Build history of the part. All positions in model axes, mm. A direction names the side the tool comes from. Give positions to 0.01 mm unless a question says otherwise; leave off trailing zeros. Order: outer loops, then holes, each group sorted by start corner. A loop starts at its lowest first (then second) coordinate and runs counter-clockwise, first axis right, second up. Notation, with made-up numbers: M -1.5,36 L 22.5,36 A31 ccw 22.5,71 Z; hole C 20,2 d1. An arc over 180 degrees is marked long. Use CSV: the item, a comma, the result in double quotes. Start each with the question number.
Item 1: Pin check, flat tip, straight feed: P1, Ø6.5, axis at x = 20.5, y = 3.5, coming from the +Z side. Stop position of the tip, or through.
Item 2: Which spindle directions (+Z, -Z, +X, -X, +Y, -Y) get a long thin tool onto all of the face, cutting with end or side? Do faces 4 (the flat face through (14, 29, 12)), 5 (the flat face through (4, 24, 7)), 6 (the cylindrical face through (-4, 38.07, 9.86)). Say none if no direction does.
Item 3: Band-saw the part on B-B on z = 16. Write the cut outline in (x, y).
Item 4: Two-plate mould, pull along Y, no slides. Class faces 1 (the flat face through (5, 26, 0)), 2 (the flat face through (14, -3, 10)), 3 (the flat face through (14, -10.5, 10)): pulls with the +Y half, pulls with the -Y half, needs draft (parallel to the pull), parting line crosses it, or undercut.
Item 5: Band-saw the part on D-D on y = 28. Write the cut outline in (x, z).
Item 6: Band-saw the part on A-A on x = 22. Write the cut outline in (y, z), plus the area to 3 significant figures.
Item 7: Wall check: line 1 along Y through (x, z) = (28.5, 17.5); line 2 along Y through (x, z) = (18, 10); line 3 along X through (y, z) = (14, 12.5). Give the ranges that are in metal, low to high.
Item 8: Band-saw the part on C-C on y = 21.5. Write the cut outline in (x, z), plus the area to 3 significant figures.
from build123d import *

# Parameters (mm, degrees)
SKETCH2_W           = 29
SKETCH2_H           = 5
BOSS_EXTRUDE2_DEPTH = 20
SKETCH3_W           = 8
SKETCH3_H           = 5
SKETCH3_W_2         = 29
SKETCH3_H_2         = 6
CUT_EXTRUDE1_DEPTH  = 5


with BuildPart() as part:
    # Sketch2 → Boss-Extrude2 (new body)
    with BuildSketch(Plane.XY):
        with BuildLine():
            ThreePointArc((-5.5, -5.5), (-4.035533906, -9.035533906), (-0.5, -10.5))
            Line((-0.5, -10.5), (29.5, -10.5))
            ThreePointArc((29.5, -10.5), (33.035533906, -9.035533906), (34.5, -5.5))
            Line((34.5, -5.5), (34.5, 34.5))
            ThreePointArc((34.5, 34.5), (33.035533906, 38.035533906), (29.5, 39.5))
            Line((29.5, 39.5), (-0.5, 39.5))
            ThreePointArc((-0.5, 39.5), (-4.035533906, 38.035533906), (-5.5, 34.5))
            Line((-5.5, 34.5), (-5.5, -5.5))
        make_face()
        Polygon((29, 6), (0, 6), (0, 24), (8, 24), (8, 29), (21, 29), (21, 24), (29, 24), align=None, mode=Mode.SUBTRACT)
        with Locations((14.5, -5.5)):
            Rectangle(SKETCH2_W, SKETCH2_H, mode=Mode.SUBTRACT)
        with Locations((14.5, 34.5)):
            Rectangle(SKETCH2_W, SKETCH2_H, mode=Mode.SUBTRACT)
    extrude(amount=BOSS_EXTRUDE2_DEPTH)

    # Sketch3 → Cut-Extrude1 (cut)
    with BuildSketch(Plane.XY.offset(20)):
        with Locations((4, 26.5)):
            Rectangle(SKETCH3_W, SKETCH3_H)
        with Locations((25, 26.5)):
            Rectangle(SKETCH3_W, SKETCH3_H)
        with Locations((14.5, 3)):
            Rectangle(SKETCH3_W_2, SKETCH3_H_2)
    extrude(amount=-CUT_EXTRUDE1_DEPTH, mode=Mode.SUBTRACT)


solid = part.part
Model answer:
1,P1,"stops at z = 15"
2,face 4,"+Z"
2,face 5,"+Z, -Z"
2,face 6,"+Z, -Z, -X, +Y"
3,outline,"M -5.5,-5.5 A5 ccw -0.5,-10.5 L 29.5,-10.5 A5 ccw 34.5,-5.5 L 34.5,34.5 A5 ccw 29.5,39.5 L -0.5,39.5 A5 ccw -5.5,34.5 Z; hole M 0,-8 L 29,-8 L 29,-3 L 0,-3 Z; hole M 0,0 L 29,0 L 29,29 L 0,29 Z; hole M 0,32 L 29,32 L 29,37 L 0,37 Z"
4,face 1,"needs draft"
4,face 2,"undercut"
4,face 3,"pulls with the -Y half"
5,outline,"M -5.5,0 L 8,0 L 8,15 L 0,15 L 0,20 L -5.5,20 Z; M 21,0 L 34.5,0 L 34.5,20 L 29,20 L 29,15 L 21,15 Z"
6,outline,"M -10.5,0 L -8,0 L -8,20 L -10.5,20 Z; M -3,0 L 6,0 L 6,15 L 0,15 L 0,20 L -3,20 Z; M 24,0 L 32,0 L 32,20 L 29,20 L 29,15 L 24,15 Z; M 37,0 L 39.5,0 L 39.5,20 L 37,20 Z"
6,area,"385 mm^2"
7,line 1,"y = -10.5 to -8, -3 to 0, 29 to 32, 37 to 39.5"
7,line 2,"y = -10.5 to -8, -3 to 6, 29 to 32, 37 to 39.5"
7,line 3,"x = -5.5 to 0, 29 to 34.5"
8,outline,"M -5.5,0 L 0,0 L 0,20 L -5.5,20 Z; M 29,0 L 34.5,0 L 34.5,20 L 29,20 Z"
8,area,"220 mm^2"
